Build history of the part. All positions in model axes, mm. Coordinates: 2 decimals unless noted, no trailing zeros. Loops run counter-clockwise (first coordinate to the right, second up) from the corner with the lowest first, then second, coordinate; pieces in that order, holes last.
(1) Slice it at A-A (z = 62.5). Give the cut face in (x, y), and give its area (3 significant figures).
(2) Wall check: L1, parallel to X at y = 1.3, z = -101; L2, parallel to Y at x = -0.65, z = -128; L3, parallel to X at y = -0.75, z = 135.5. Give the ranges that are in metal, low to high.
(3) Flat gauge pins, fed straight in: P1, Ø2, axis at x = 2, z = 0.5, coming from the +Y side; P2, Ø3, axis at x = -1.5, z = 121.5, coming from the +Y side. Where does each tip first touch, or does it go through?
from build123d import *

# Parameters (mm, degrees)
SKETCH3_R           = 3
BOSS_EXTRUDE1_DEPTH = 152.4
CHAMFER1_SIZE       = 0.3
FILLET1_R           = 0.225


with BuildPart() as part:
    # Sketch3 → Boss-Extrude1 (new, symmetric)
    with BuildSketch(Plane.XY):
        with Locations(Location((0, 0, 0), (0, 0, 180))):
            Circle(SKETCH3_R)
    extrude(amount=BOSS_EXTRUDE1_DEPTH, both=True)

    # Chamfer1
    chamfer1_edges = [part.edges().sort_by_distance(p)[0] for p in [
        (3, 0, -152.4),
        (3, 0, 152.4),
    ]]
    chamfer(chamfer1_edges, length=CHAMFER1_SIZE)

    # Fillet1
    fillet1_edges = [part.edges().sort_by_distance(p)[0] for p in [
        (3, 0, 152.1),
        (3, 0, -152.1),
    ]]
    fillet(fillet1_edges, radius=FILLET1_R)


solid = part.part
Response values:
1. outline: circle Ø6 at (0, 0)
1. area: 28.3 mm2
2. L1: x = -2.7 to 2.7
2. L2: y = -2.93 to 2.93
2. L3: x = -2.9 to 2.9
3. P1: stops at y = 2.83
3. P2: stops at y = 3
